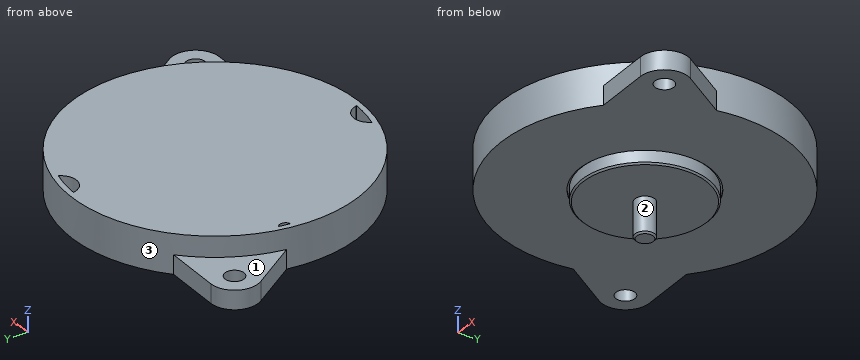
from build123d import *

# Parameters (mm, degrees)
SKETCH4_R           = 18.2
BOSS_EXTRUDE3_DEPTH = 5
CUT_EXTRUDE2_DEPTH  = 2
SKETCH6_R           = 1.2
BOSS_EXTRUDE4_DEPTH = 2.4
SKETCH1_R           = 8.25
CUT_EXTRUDE1_DEPTH  = 0.2
SKETCH2_R           = 8
BOSS_EXTRUDE1_DEPTH = 1.7
SKETCH3_R           = 1.25
BOSS_EXTRUDE2_DEPTH = 4.5
CHAMFER1_SIZE       = 0.2
CHAMFER2_SIZE       = 0.2


with BuildPart() as part:
    # Sketch4 → Boss-Extrude3 (new body)
    with BuildSketch(Plane.XY):
        Circle(SKETCH4_R)
    extrude(amount=BOSS_EXTRUDE3_DEPTH)

    # Sketch5 → Cut-Extrude2 (cut)
    with BuildSketch(Plane.XY.offset(5)):
        with BuildLine():
            ThreePointArc((1.322526628, 17.302811533), (2.918295178, 15.731610002), (4.971429117, 16.625921213))
            ThreePointArc((4.971429117, 16.625921213), (5.071370491, 16.706466919), (5.199688837, 16.709674922))
            ThreePointArc((5.199688837, 16.709674922), (3.191885351, 17.20644844), (1.139493871, 17.462862128))
            ThreePointArc((1.139493871, 17.462862128), (1.258123981, 17.413843908), (1.322526628, 17.302811533))
        make_face()
        with BuildLine():
            ThreePointArc((-17.208763457, 2.536145077), (-16.729701345, 3.103446294), (-16.97341649, 3.804826439))
            ThreePointArc((-16.97341649, 3.804826439), (-17.032179911, 3.894218363), (-17.036464522, 4.001109419))
            ThreePointArc((-17.036464522, 4.001109419), (-17.20644844, 3.191885351), (-17.338016995, 2.375535034))
            ThreePointArc((-17.338016995, 2.375535034), (-17.295679076, 2.473777369), (-17.208763457, 2.536145077))
        make_face()
        with BuildLine():
            ThreePointArc((-5.199688837, -16.709674922), (-3.191885351, -17.20644844), (-1.139493871, -17.462862128))
            ThreePointArc((-1.139493871, -17.462862128), (-1.258123981, -17.413843908), (-1.322526628, -17.302811533))
            ThreePointArc((-1.322526628, -17.302811533), (-2.918295178, -15.731610002), (-4.971429117, -16.625921213))
            ThreePointArc((-4.971429117, -16.625921213), (-5.071370491, -16.706466919), (-5.199688837, -16.709674922))
        make_face()
    extrude(amount=-CUT_EXTRUDE2_DEPTH, mode=Mode.SUBTRACT)

    # Sketch6 → Boss-Extrude4 (add)
    # profile 1 of 2: a face of its own
    with BuildSketch(Plane.XY):
        with BuildLine():
            Line((-19.06335062, 14.072551336), (-11.880431968, 13.787506527))
            ThreePointArc((-11.880431968, 13.787506527), (-15.761662349, 9.1), (-17.880546892, 3.395002629))
            Line((-17.880546892, 3.395002629), (-21.718862263, 9.47307025))
            ThreePointArc((-21.718862263, 9.47307025), (-21.78038431, 12.574910744), (-19.06335062, 14.072551336))
        make_face()
        with Locations((-19.182308099, 11.074910744)):
            Circle(SKETCH6_R, mode=Mode.SUBTRACT)
    # profile 2 of 2: a face of its own
    with BuildSketch(Plane.XY):
        with BuildLine():
            Line((17.880546892, -3.395002629), (21.718862263, -9.47307025))
            ThreePointArc((21.718862263, -9.47307025), (21.78038431, -12.574910744), (19.06335062, -14.072551336))
            Line((19.06335062, -14.072551336), (11.880431968, -13.787506527))
            ThreePointArc((11.880431968, -13.787506527), (15.761662349, -9.1), (17.880546892, -3.395002629))
        make_face()
        with Locations((19.182308099, -11.074910744)):
            Circle(SKETCH6_R, mode=Mode.SUBTRACT)
    extrude(amount=BOSS_EXTRUDE4_DEPTH)

    # Sketch1 → Cut-Extrude1 (cut)
    with BuildSketch(Plane(origin=(0, 0, 0), x_dir=(-1, 0, 0), z_dir=(0, 0, -1))):
        with Locations(Location((0, 0, 0), (0, 0, 180))):
            Circle(SKETCH1_R)
    extrude(amount=-CUT_EXTRUDE1_DEPTH, mode=Mode.SUBTRACT)

    # Sketch2 → Boss-Extrude1 (add)
    with BuildSketch(Plane(origin=(0, 0, 0.2), x_dir=(-1, 0, 0), z_dir=(0, 0, -1))):
        with Locations(Location((0, 0, 0), (0, 0, 180))):
            Circle(SKETCH2_R)
    extrude(amount=BOSS_EXTRUDE1_DEPTH)

    # Sketch3 → Boss-Extrude2 (add)
    with BuildSketch(Plane(origin=(0, 0, -1.5), x_dir=(-1, 0, 0), z_dir=(0, 0, -1))):
        Circle(SKETCH3_R)
    extrude(amount=BOSS_EXTRUDE2_DEPTH)

    # Chamfer1
    chamfer1_edges = [part.edges().sort_by_distance(p)[0] for p in [
        (1.25, 0, -6),
    ]]
    chamfer(chamfer1_edges, length=CHAMFER1_SIZE)

    # Chamfer2
    chamfer2_edges = [part.edges().sort_by_distance(p)[0] for p in [
        (-8, 0, -1.5),
    ]]
    chamfer(chamfer2_edges, length=CHAMFER2_SIZE)


solid = part.part
Model file for the job. Use its own axes, mm. Face numbers are marked on the shaded views. A direction names the side the tool comes from. Give positions to 0.01 mm unless a question says otherwise; leave off trailing zeros. Order: outer loops, then holes, each group sorted by start corner. A loop starts at its lowest first (then second) coordinate and runs counter-clockwise, first axis right, second up. Notation, with made-up numbers: M 4.25,54 L 43.25,54 A31 cw 43.25,85 Z; hole C 31.25,38.5 d1. An arc over 180 degrees is marked long. Put each result on its own line as item: value. Start each with the question number.
(1) Band-saw the part on B-B on z = 0.75. Give the cut face in (x, y) (1 decimal), then the cut area to 3 significant figures.
(2) Pin check, flat tips, straight feed: pin 1 Ø1 at (x, z) = (-5.5, -1.5) entering from -Y; pin 2 Ø3 at (x, z) = (13, 0.5) entering from -Y; pin 3 Ø3 at (x, y) = (19.18, -11.07) entering from -Z. Stop position of each tip, or through.
(3) Drill centre lines: L1, parallel to Y at x = 0, z = 0.1; L2, parallel to Z at x = -11.5, y = 10; L3, parallel to X at y = -16, z = 3.75. Where is each one in solid material? Low to high. Write a range as [from, to].
(4) Band-saw the part on A-A on y = 0. Give the cut face in (x, z), then the cut area to 3 significant figures.
(5) Tool access for the marked faces 1, 2 and 3: list every direction of +Z, -Z, +X, -X, +Y, -Y with a clear straight run to the whole face (end or side of a thin tool).
(6) Band-saw the part on D-D on z = -3. Give the cut face in (x, y), then the cut area to 3 significant figures.
Results below:
1. outline: M -21.7,9.5 L -17.9,3.4 A18.2 ccw 11.9,-13.8 L 19.1,-14.1 A3 ccw 21.7,-9.5 L 17.9,-3.4 A18.2 ccw -11.9,13.8 L -19.1,14.1 A3 ccw Z; hole C -19.2,11.1 d2.4; hole C 19.2,-11.1 d2.4
1. area: 1,140 mm2
2. pin 1: stops at y = -6.21
2. pin 2: stops at y = -14.11
2. pin 3: stops at z = 0
3. L1: y = [-18.2, -8.25], [-8, 8], [8.25, 18.2]
3. L2: z = [0, 5]
3. L3: x = [-8.67, -4.34], [-2.23, 8.67]
4. outline: M -18.2,0 L -8.25,0 L -8.25,0.2 L -8,0.2 L -8,-1.3 L -7.8,-1.5 L -1.25,-1.5 L -1.25,-5.8 L -1.05,-6 L 1.05,-6 L 1.25,-5.8 L 1.25,-1.5 L 7.8,-1.5 L 8,-1.3 L 8,0.2 L 8.25,0.2 L 8.25,0 L 18.2,0 L 18.2,5 L -18.2,5 Z
4. area: 217 mm2
5. face 1: +Z, -X, +Y
5. face 2: -Z
5. face 3: +Z
6. outline: C 0,0 d2.5
6. area: 4.91 mm2
